CAD build for the part. Positions are in the model's coordinates, mm. A direction names the side the tool comes from. Give positions to 0.01 mm unless a question says otherwise; leave off trailing zeros. Write each loop counter-clockwise with the first axis right and the second up, starting at its lowest first coordinate (ties: lowest second). Pieces come first, ordered by that corner, then holes. Notation, with made-up numbers: (-17.75, -27) - (23.25, -27) arc R8 cw to (23.25, -22) - close; hole circle Ø11 at (43.25, 72). An arc over 180 degrees is marked (long way). Answer as a JSON object with one key per item and string values.
from build123d import *

# Parameters (mm, degrees)
SKETCH007_W                   = 2.25
SKETCH007_H                   = 5.4
POCKET003_DEPTH               = 3
POCKET003_MIRRORED001_2_DEPTH = 3


with BuildPart() as part:
    # Sketch007 → Revolution (revolve)
    with BuildSketch(Plane.YZ):
        with Locations((1.125, 2.7)):
            Rectangle(SKETCH007_W, SKETCH007_H)
    revolve(axis=Axis((0, 0, 0), (0, 0, 1)))

    # Sketch008 → Pocket003 (cut)
    with BuildSketch(Plane.XY):
        Polygon((-3, 0), (0, 0), (0, 1.2), (-1.2, 1.2), (-1.2, 0.5), (-3, 0.5), align=None)
    pocket003 = extrude(amount=POCKET003_DEPTH, mode=Mode.SUBTRACT)

    # Sketch008 Mirrored001 2 → Pocket003 Mirrored001 2 (cut)
    with BuildSketch(Plane(origin=(0, 0, 0), x_dir=(-1, 0, 0), z_dir=(0, 0, -1))):
        Polygon((-3, 0), (0, 0), (0, 1.2), (-1.2, 1.2), (-1.2, 0.5), (-3, 0.5), align=None)
    pocket003_mirrored001_2 = extrude(amount=-POCKET003_MIRRORED001_2_DEPTH, mode=Mode.SUBTRACT)

    # Mirrored002: Pocket003, Pocket003 Mirrored001 2 across Sketch008 H_Axis
    add(pocket003.mirror(Plane.ZX), mode=Mode.SUBTRACT)
    add(pocket003_mirrored001_2.mirror(Plane.ZX), mode=Mode.SUBTRACT)


with BuildPart() as part_1:
    # Body003 placement: moved
    add(part.part.moved(Location((80.72, -163.91, 16.2))))


solid = part_1.part
Item 1: Probe line 1 (Z direction, x = 80.85, y = -164.4); line 2 (X direction, y = -163.3, z = 17.45); line 3 (X direction, y = -164.65, z = 17.4). List the from-to ranges inside material, lowest first. Write a range as from..to.
Entries:
{"line 1": "19.2..21.6", "line 2": "78.55..79.52, 81.92..82.89", "line 3": "78.6..79.52, 81.92..82.84"}
Item 2: Mould opens along X. For faces 4 (the flat face through (81, -165.11, 18)), 5 (the cylindrical face through (80.044, -161.764, 18.938)), 6 (the flat face through (82.4, -164.41, 17.7)) say: +X half, -X half, draft (parallel to the pull), parting line (faces both ways), or undercut.
Entries:
{"face 4": "undercut", "face 5": "parting line", "face 6": "draft"}
Item 3: Cut at C-C (y = -163.05). Give the cut face in (x, z), and give its area (3 significant figures).
Entries:
{"outline": "(78.64, 16.2) - (79.52, 16.2) - (79.52, 19.2) - (81.92, 19.2) - (81.92, 16.2) - (82.8, 16.2) - (82.8, 21.6) - (78.64, 21.6) - close", "area": "15.3 mm2"}
Item 4: Cut at A-A (z = 19.05). Give the cut face in (x, y).
Entries:
{"outline": "(78.53, -164.41) arc R2.25 ccw to (82.91, -164.41) - (81.92, -164.41) - (81.92, -165.11) - (79.52, -165.11) - (79.52, -164.41) - close; (78.53, -163.41) - (79.52, -163.41) - (79.52, -162.71) - (81.92, -162.71) - (81.92, -163.41) - (82.91, -163.41) arc R2.25 ccw to start"}
Item 5: Cut at B-B (x = 80.72). Give the cut face in (y, z), and give its area (3 significant figures).
Entries:
{"outline": "(-166.16, 16.2) - (-165.11, 16.2) - (-165.11, 19.2) - (-162.71, 19.2) - (-162.71, 16.2) - (-161.66, 16.2) - (-161.66, 21.6) - (-166.16, 21.6) - close", "area": "17.1 mm2"}
Item 6: Which spindle directions (+Z, -Z, +X, -X, +Y, -Y) get a long thin tool onto all of the face, cutting with end or side? Do faces 1 (the flat face through (81, -162.71, 18)), 2 (the flat face through (80.7, -162.5, 16.2)), 3 (the flat face through (82.4, -163.41, 17.7)). Say none if no direction does.
Entries:
{"face 1": "-Z", "face 2": "-Z, +X, -X, +Y, -Y", "face 3": "-Z, +X, -X"}
Item 7: Cut at D-D (z = 21.2). Give the cut face in (x, y), and give its area (3 significant figures).
Entries:
{"outline": "circle Ø4.5 at (80.72, -163.91)", "area": "15.9 mm2"}
Item 8: Flat gauge pins, fed straight in: P1, Ø0.8, axis at x = 82.5, z = 17.5, coming from the -Y side; P2, Ø1.1, axis at x = 79, z = 18.5, coming from the +Y side; P3, Ø0.6, axis at y = -163, z = 17.5, coming from the +X side; P4, Ø2, axis at y = -163, z = 19.5, coming from the -X side. Where does each tip first touch, or does it go through?
Entries:
{"P1": "y = -165.69", "P2": "y = -161.99", "P3": "x = 82.89", "P4": "x = 78.47"}
